Geometry check sheet. Reference: the model listing, model coordinates, mm. A direction names the side the tool comes from. Coordinates: 2 decimals unless noted, no trailing zeros. Loops run counter-clockwise (first coordinate to the right, second up) from the corner with the lowest first, then second, coordinate; pieces in that order, holes last. Notation, with made-up numbers: (34, 7.5) - (79, 7.5) arc R29 cw to (79, 31.5) - close; hole circle Ø8 at (4.25, 35.5). An arc over 180 degrees is marked (long way). Write each question's results on one line, items separated by ' | '. Start each with the question number.
(1) Material ranges on probe 1 along Z at (x, y) = (6.5, 7); probe 2 along Y at (x, z) = (0.5, 0.75); probe 3 along Y at (x, z) = (-17, 1), recorded low to high.
(2) Access from +Z, -Z, +X, -X, +Y, -Y to the whole of each face (thin tool, end or side, straight path). Record for faces 4 (the face through (-15.86, -11.9, -1.77)), 5 (the face through (5.82, 10.75, 3.27)), 6 (the face through (-20, -11, -2)).
(3) Sectioned sample at C-C (y = 9). Enter the section's corners in (x, z).
(4) Sectioned sample at D-D (x = 1.5). Enter the section's corners in (y, z), plus the area to 3 significant figures.
(5) Sectioned sample at A-A (z = -1.5). Enter the section's corners in (x, y).
(6) Go/stop test with flat-tipped pins: pin 1 Ø2 at (x, y) = (4.5, -4.5) entering from -Z; pin 2 Ø12 at (x, y) = (-15, -4.5) entering from +Z; pin 3 Ø2 at (x, z) = (19, 0.5) entering from -Y. Record where each tip stops, or that it passes through.
(7) Sectioned sample at B-B (y = 1). Enter the section's corners in (x, z), plus the area to 3 significant figures.
(8) Mould release check, pull along Y, two halves, no side actions. Record for faces 1 (the face through (2.43, -3.06, 3.27)), 2 (the face through (15, -16, -2)), 3 (the face through (15.86, -11.9, -1.77)): pulls with the +Y half, pulls with the -Y half, needs draft (parallel to the pull), parting line crosses it, or undercut.
from build123d import *

# Parameters (mm, degrees)
SKETCH1_W                                        = 46
SKETCH1_H                                        = 36
BOSS_EXTRUDE1_DEPTH                              = 4.5
SKETCH2_W                                        = 8
SKETCH2_H                                        = 7
BOSS_EXTRUDE2_DEPTH                              = 3.5
SKETCH3_W                                        = 7.999999995
SKETCH3_H                                        = 7
BOSS_EXTRUDE3_DEPTH                              = 3.5
SKETCH4_W                                        = 4
SKETCH4_H                                        = 3
F_1_7_1_7_DIAMETER_HOLE1_D                       = 1.7
F_1_7_1_7_DIAMETER_HOLE1_DEPTH                   = 7
F_1_7_1_7_DIAMETER_HOLE1_TIP                     = 0.510731526
F_2_5_2_5_DIAMETER_HOLE1_D                       = 2.5
F_2_5_2_5_DIAMETER_HOLE1_DEPTH                   = 6
F_2_5_2_5_DIAMETER_HOLE1_TIP                     = 0.751075774
HOLE1_D                                          = 10.4
HOLE1_CBORE_D                                    = 12.2
HOLE1_CBORE_DEPTH                                = 3.3
CBORE_FOR_M3_HEX_HEAD_MACHINE_SCREW1_D           = 3.2
CBORE_FOR_M3_HEX_HEAD_MACHINE_SCREW1_DEPTH       = 8.000025
CBORE_FOR_M3_HEX_HEAD_MACHINE_SCREW1_CBORE_D     = 5.4
CBORE_FOR_M3_HEX_HEAD_MACHINE_SCREW1_CBORE_DEPTH = 2.5
F_4_2_4_2_DIAMETER_HOLE1_D                       = 4.2
F_4_2_4_2_DIAMETER_HOLE1_DEPTH                   = 7
FILLET1_R                                        = 3
FILLET2_R                                        = 8


with BuildPart() as part:
    # Sketch1 → Boss-Extrude1 (new body)
    with BuildSketch(Plane.XY.offset(4.5)):
        Rectangle(SKETCH1_W, SKETCH1_H)
    extrude(amount=-BOSS_EXTRUDE1_DEPTH)

    # Sketch2 → Boss-Extrude2 (add)
    with BuildSketch(Plane(origin=(0, 0, 0), x_dir=(-1, 0, 0), z_dir=(0, 0, -1))):
        with Locations((-19, -14.5)):
            Rectangle(SKETCH2_W, SKETCH2_H)
    extrude(amount=BOSS_EXTRUDE2_DEPTH)

    # Sketch3 → Boss-Extrude3 (add)
    with BuildSketch(Plane(origin=(0, 0, 0), x_dir=(-1, 0, 0), z_dir=(0, 0, -1))):
        with Locations((19.000000003, -14.5)):
            Rectangle(SKETCH3_W, SKETCH3_H)
    extrude(amount=BOSS_EXTRUDE3_DEPTH)

    # Sketch4 → Revolve1 (revolve)
    with BuildSketch(Plane.XZ.offset(2)):
        with Locations((-3, 6)):
            Rectangle(SKETCH4_W, SKETCH4_H)
    revolve(axis=Axis((-5, -2, 7.5), (0, 0, -1)))

    # Ø1.7 (1.7) Diameter Hole1
    with Locations(Plane(origin=(0, -18, 0), x_dir=(-1, 0, 0), z_dir=(0, -1, 0))):
        with Locations((0, -2.25)):
            Hole(F_1_7_1_7_DIAMETER_HOLE1_D / 2, depth=F_1_7_1_7_DIAMETER_HOLE1_DEPTH)
            with Locations((0, 0, -(F_1_7_1_7_DIAMETER_HOLE1_DEPTH + F_1_7_1_7_DIAMETER_HOLE1_TIP / 2))):  # 118° drill point
                Cone(0, F_1_7_1_7_DIAMETER_HOLE1_D / 2, F_1_7_1_7_DIAMETER_HOLE1_TIP, mode=Mode.SUBTRACT)

    # Ø2.5 (2.5) Diameter Hole1
    with Locations(Plane(origin=(0, -18, 0), x_dir=(-1, 0, 0), z_dir=(0, -1, 0))):
        with Locations((-19, -0.5), (19, -0.5)):
            Hole(F_2_5_2_5_DIAMETER_HOLE1_D / 2, depth=F_2_5_2_5_DIAMETER_HOLE1_DEPTH)
            with Locations((0, 0, -(F_2_5_2_5_DIAMETER_HOLE1_DEPTH + F_2_5_2_5_DIAMETER_HOLE1_TIP / 2))):  # 118° drill point
                Cone(0, F_2_5_2_5_DIAMETER_HOLE1_D / 2, F_2_5_2_5_DIAMETER_HOLE1_TIP, mode=Mode.SUBTRACT)

    # Hole1 (through all)
    with Locations(Plane(origin=(0, 0, 0), x_dir=(-1, 0, 0), z_dir=(0, 0, -1))):
        with Locations((0.645780782, 5.541728913)):
            CounterBoreHole(HOLE1_D / 2, HOLE1_CBORE_D / 2, HOLE1_CBORE_DEPTH)

    # CBORE for M3 Hex Head Machine Screw1
    with Locations(Plane.XY.offset(4.5)):
        with Locations((0.980122741, -5.337445584), (7.962908944, 12.389389916), (-10.88037403, 9.573242407)):
            CounterBoreHole(CBORE_FOR_M3_HEX_HEAD_MACHINE_SCREW1_D / 2, CBORE_FOR_M3_HEX_HEAD_MACHINE_SCREW1_CBORE_D / 2, CBORE_FOR_M3_HEX_HEAD_MACHINE_SCREW1_CBORE_DEPTH, depth=CBORE_FOR_M3_HEX_HEAD_MACHINE_SCREW1_DEPTH)

    # Ø4.2 (4.2) Diameter Hole1
    with Locations(Plane.XY.offset(7.5)):
        with Locations((-5, -2)):
            Hole(F_4_2_4_2_DIAMETER_HOLE1_D / 2, depth=F_4_2_4_2_DIAMETER_HOLE1_DEPTH)

    # Fillet1
    fillet1_edges = [part.edges().sort_by_distance(p)[0] for p in [
        (-15.000000005, -11, -1.75),
        (15, -11, -1.75),
    ]]
    fillet(fillet1_edges, radius=FILLET1_R)

    # Fillet2
    fillet2_edges = [part.edges().sort_by_distance(p)[0] for p in [
        (-23, 18, 2.25),
        (23, 18, 2.25),
    ]]
    fillet(fillet2_edges, radius=FILLET2_R)


solid = part.part
Outcome:
1) probe 1: z = 0 to 4.5 | probe 2: y = -18 to -6.86, -3.81 to -0.45, 11.53 to 18 | probe 3: y = -18 to 17.75
2) face 4: -Z, +Y | face 5: +Z | face 6: -Z, +X, -X, +Y
3) outline: (-23, 0) - (-12.37, 0) - (-12.37, 2) - (-13.52, 2) - (-13.52, 4.5) - (-23, 4.5) - close; (-9.39, 0) - (-5.67, 0) - (-5.67, 3.3) - (-4.53, 3.3) - (-4.53, 4.5) - (-8.24, 4.5) - (-8.24, 2) - (-9.39, 2) - close; (3.24, 3.3) - (4.38, 3.3) - (4.38, 0) - (23, 0) - (23, 4.5) - (3.24, 4.5) - close
4) outline: (-18, 0) - (-6.85, 0) - (-6.85, 2) - (-7.99, 2) - (-7.99, 4.5) - (-18, 4.5) - close; (-3.82, 0) - (-0.17, 0) - (-0.17, 3.3) - (0.81, 3.3) - (0.81, 4.5) - (-2.69, 4.5) - (-2.69, 2) - (-3.82, 2) - close; (10.28, 3.3) - (11.25, 3.3) - (11.25, 0) - (18, 0) - (18, 4.5) - (10.28, 4.5) - close | area: 93.6 mm2
5) outline: (-23, -18) - (-15, -18) - (-15, -14) arc R3 ccw to (-18, -11) - (-23, -11) - close; (15, -18) - (23, -18) - (23, -11) - (18, -11) arc R3 ccw to (15, -14) - close
6) pin 1: stops at z = 0 | pin 2: stops at z = 4.5 | pin 3: stops at y = -11.85
7) outline: (-23, 0) - (-4.72, 0) - (-4.72, 3.3) - (-3.18, 3.3) - (-3.18, 7.5) - (-7.65, 7.5) - (-7.65, 4.5) - (-23, 4.5) - close; (1.89, 3.3) - (3.43, 3.3) - (3.43, 0) - (23, 0) - (23, 4.5) - (1.89, 4.5) - close | area: 187 mm2
8) face 1: undercut | face 2: needs draft | face 3: pulls with the +Y half
